```python
from build123d import *

# Parameters (mm, degrees)
SKETCH_1_W          = 120
SKETCH_1_H          = 35
EXTRUDE_1_DEPTH     = 3
SKETCH_2_W          = 30
SKETCH_2_H          = 17
CUT_EXTRUDE_1_DEPTH = 63.571958576
SKETCH_3_R          = 1.3
CUT_EXTRUDE_2_DEPTH = 63.571958576
SKETCH_4_R          = 1.4
CUT_EXTRUDE_3_DEPTH = 63.571958576
SKETCH_5_W          = 10
SKETCH_5_H          = 5
CUT_EXTRUDE_4_DEPTH = 63.571958576
CHAMFER_1_SIZE      = 4
CHAMFER_1_SIZE2     = 8.578027682
CHAMFER_2_SIZE      = 4
CHAMFER_2_SIZE2     = 8.578027682
FILLET_1_R          = 5
CHAMFER_3_SIZE      = 4


with BuildPart() as part:
    # 草图1 → 凸台-拉伸1 (new body)
    with BuildSketch(Plane(origin=(0, 0, 0), x_dir=(1, 0, 0), z_dir=(0, 1, 0))):
        Rectangle(SKETCH_1_W, SKETCH_1_H)
    extrude(amount=EXTRUDE_1_DEPTH)

    # 草图2 → 切除-拉伸1 (cut, through all)
    with BuildSketch(Plane(origin=(0, 3, 0), x_dir=(1, 0, 0), z_dir=(0, 1, 0))):
        with Locations((0, 9)):
            Rectangle(SKETCH_2_W, SKETCH_2_H)
    extrude(amount=-CUT_EXTRUDE_1_DEPTH, mode=Mode.SUBTRACT)

    # 草图3 → 切除-拉伸2 (cut, through all)
    with BuildSketch(Plane(origin=(0, 3, 0), x_dir=(1, 0, 0), z_dir=(0, 1, 0))):
        with Locations(Location((-57, 12.5, 0), (0, 0, 270))):
            Circle(SKETCH_3_R)
        with Locations(Location((-57, -7.5, 0), (0, 0, 270))):
            Circle(SKETCH_3_R)
        with Locations(Location((57, -7.5, 0), (0, 0, 90))):
            Circle(SKETCH_3_R)
        with Locations(Location((57, 12.5, 0), (0, 0, 90))):
            Circle(SKETCH_3_R)
    extrude(amount=-CUT_EXTRUDE_2_DEPTH, mode=Mode.SUBTRACT)

    # 草图4 → 切除-拉伸3 (cut, through all)
    with BuildSketch(Plane(origin=(0, 3, 0), x_dir=(1, 0, 0), z_dir=(0, 1, 0))):
        with Locations(Location((5.4, -9.5, 0), (0, 0, 270))):
            Circle(SKETCH_4_R)
        with Locations(Location((20.15, -9.5, 0), (0, 0, 270))):
            Circle(SKETCH_4_R)
        with Locations(Location((27.4, -9.5, 0), (0, 0, 270))):
            Circle(SKETCH_4_R)
        with Locations(Location((42.15, -9.5, 0), (0, 0, 270))):
            Circle(SKETCH_4_R)
        with Locations(Location((-1.85, -9.5, 0), (0, 0, 270))):
            Circle(SKETCH_4_R)
        with Locations(Location((-16.6, -9.5, 0), (0, 0, 270))):
            Circle(SKETCH_4_R)
        with Locations(Location((-23.85, -9.5, 0), (0, 0, 270))):
            Circle(SKETCH_4_R)
        with Locations(Location((-38.6, -9.5, 0), (0, 0, 270))):
            Circle(SKETCH_4_R)
    extrude(amount=-CUT_EXTRUDE_3_DEPTH, mode=Mode.SUBTRACT)

    # 草图5 → 切除-拉伸4 (cut, through all)
    with BuildSketch(Plane(origin=(0, 3, 0), x_dir=(1, 0, 0), z_dir=(0, 1, 0))):
        with Locations((-30, 7.5)):
            Rectangle(SKETCH_5_W, SKETCH_5_H)
        with Locations((30, 7.5)):
            Rectangle(SKETCH_5_W, SKETCH_5_H)
    extrude(amount=-CUT_EXTRUDE_4_DEPTH, mode=Mode.SUBTRACT)

    # 倒角1
    chamfer_1_edges = [part.edges().sort_by_distance(p)[0] for p in [
        (-15, 1.5, -17.5),
    ]]
    chamfer_1_side = [part.faces().sort_by_distance(p)[0] for p in [
        (-37.5, 1.5, -17.5),
    ]]
    chamfer(chamfer_1_edges, length=CHAMFER_1_SIZE, length2=CHAMFER_1_SIZE2, reference=chamfer_1_side[0])

    # 倒角2
    chamfer_2_edges = [part.edges().sort_by_distance(p)[0] for p in [
        (15, 1.5, -17.5),
    ]]
    chamfer_2_side = [part.faces().sort_by_distance(p)[0] for p in [
        (37.5, 1.5, -17.5),
    ]]
    chamfer(chamfer_2_edges, length=CHAMFER_2_SIZE, length2=CHAMFER_2_SIZE2, reference=chamfer_2_side[0])

    # 圆角1
    fillet_1_edges = [part.edges().sort_by_distance(p)[0] for p in [
        (-15, 1.5, -0.5),
        (15, 1.5, -0.5),
    ]]
    fillet(fillet_1_edges, radius=FILLET_1_R)

    # 倒角3
    chamfer_3_edges = [part.edges().sort_by_distance(p)[0] for p in [
        (60, 1.5, 17.5),
        (-60, 1.5, 17.5),
    ]]
    chamfer(chamfer_3_edges, length=CHAMFER_3_SIZE)


solid = part.part
```
Geometry: final body of the model. Coordinates: model frame, mm. A direction names the side the tool comes from. Round coordinates to 2 decimals unless told otherwise and drop trailing zeros. Write each loop counter-clockwise with the first axis right and the second up, starting at its lowest first coordinate (ties: lowest second). Pieces come first, ordered by that corner, then holes. Notation, with made-up numbers: (-17, 36) -> (15, 36) arc R21 cw to (15, 68) -> close; hole circle Ø7 at (10, 33.5). An arc over 180 degrees is marked (long way). Use CSV: the item, a comma, the result in double quotes. Start each with the question number.
Q1. Reachability of faces 1 (the face through (30, 2, -5)), 2 (the face through (-1, 1, 17.5)), 3 (the face through (16.97, 1.52, -13.15)) from +Z, -Z, +X, -X, +Y, -Y: full face, straight path, thin tool, end or side. Return the list, or none.
Q2. Section A-A (x = 5.4). Return loops of the section in (y, z), plus the area to 3 significant figures.
Q3. Section C-C (x = 27.4). Return loops of the section in (y, z), plus the area to 3 significant figures.
Q4. Section D-D (z = -15). Return loops of the section in (x, y).
Q5. First-contact query: pin 1 Ø0.9 at (x, y) = (-4.5, 1) entering from -Z. Flat tip, straight axial feed; report the tip coordinate or a pass-through.
Q6. Section B-B (y = 0.65). Give the number of separate pieces and of enclosed holes in the cut face, plus the area to 3 significant figures.
Q7. Line query: L1, parallel to X at y = 0.2, z = -7.5; L2, parallel to Z at x = -2, y = 0.9; L3, parallel to X at y = 0.9, z = -12.5. Output: solid intervals per line, ascending.
Result sheet:
1,face 1,"+Y, -Y"
1,face 2,"+Z, +X, -X, +Y, -Y"
1,face 3,"-Z, +Y, -Y"
2,outline,"(0, -0.5) -> (3, -0.5) -> (3, 8.1) -> (0, 8.1) -> close; (0, 10.9) -> (3, 10.9) -> (3, 17.5) -> (0, 17.5) -> close"
2,area,"45.6 mm²"
3,outline,"(0, -17.5) -> (3, -17.5) -> (3, -10) -> (0, -10) -> close; (0, -5) -> (3, -5) -> (3, 8.1) -> (0, 8.1) -> close; (0, 10.9) -> (3, 10.9) -> (3, 17.5) -> (0, 17.5) -> close"
3,area,"81.6 mm²"
4,outline,"(-60, 0) -> (-17.83, 0) -> (-17.83, 3) -> (-60, 3) -> close; (17.83, 0) -> (60, 0) -> (60, 3) -> (17.83, 3) -> close"
5,pin 1,"z = -0.5"
6,separate pieces,"1"
6,enclosed holes,"14"
6,area,"3,480 mm²"
7,L1,"-60 to -35, -25 to -15, 15 to 25, 35 to 60"
7,L2,"-0.5 to 8.11, 10.89 to 17.5"
7,L3,"-60 to -58.3, -55.7 to -16.67, 16.67 to 55.7, 58.3 to 60"
